Check sheet for the drawn part. Datum: minimum x, y, z corner. Units: mm. Round coordinates to 2 decimals unless told otherwise and drop trailing zeros. Order: outer loops, then holes, each group sorted by start corner. A loop starts at its lowest first (then second) coordinate and runs counter-clockwise, first axis right, second up. Notation, with made-up numbers: (-1, 7) -> (56, 7) arc R31 ccw to (56, 45) -> close; hole circle Ø4 at (30.5, -8.75). An arc over 180 degrees is marked (long way). Use CSV: the item, a comma, the result in double quotes.
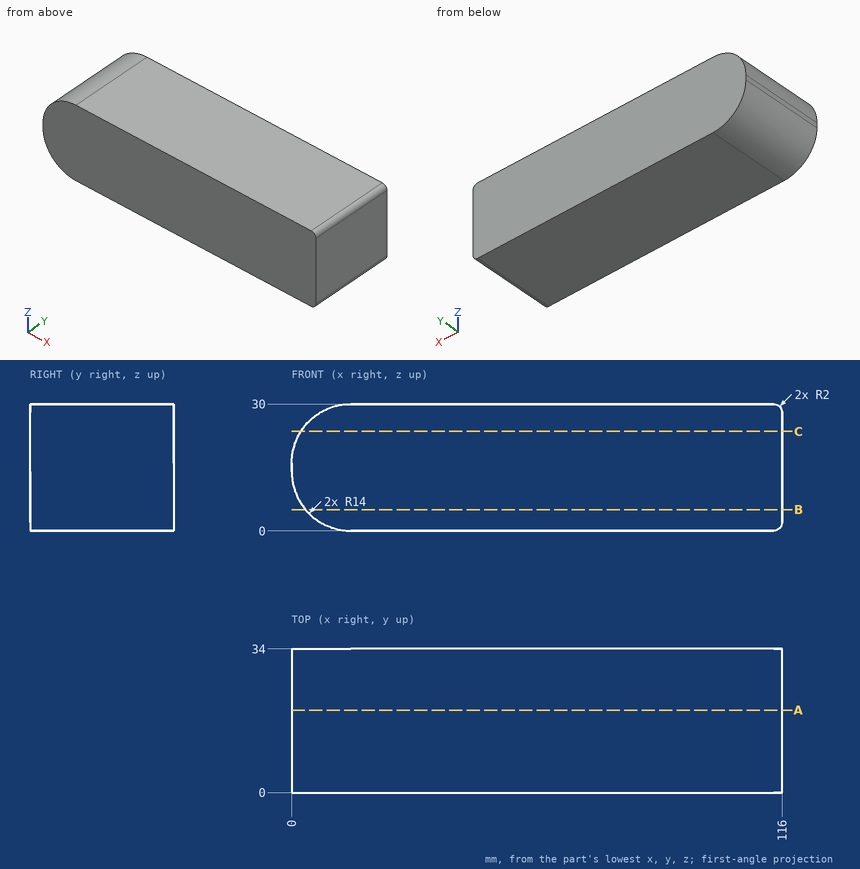
Q1. Scan lines: L1, parallel to X at y = 14.5, z = 17; L2, parallel to X at y = 12.5, z = 6; L3, parallel to Z at x = 10.5, y = 20.5. Record each from-to range of solid material in increasing order.
Result sheet:
L1,"x = 0.04 to 116"
L2,"x = 2.51 to 116"
L3,"z = 0.44 to 29.56"
Q2. Go/stop test with flat-tipped pins: pin 1 (4 mm diameter, centred on y = 12.5, z = 10.5, fed in from -X); pin 2 (4 mm diameter, centred on y = 25, z = 25, fed in from -X). Record where each tip stops, or that it passes through.
Result sheet:
pin 1,"stops at x = 0.08"
pin 2,"stops at x = 1.88"
Q3. Sectioned sample at A-A, the plane y = 19.5. Enter the section's corners in (x, z).
Result sheet:
outline,"(0, 14) arc R14 ccw to (14, 0) -> (114, 0) arc R2 ccw to (116, 2) -> (116, 28) arc R2 ccw to (114, 30) -> (14, 30) arc R14 ccw to (0, 16) -> close"
Q4. Sectioned sample at C-C, the plane z = 23.5. Enter the section's corners in (x, y).
Result sheet:
outline,"(2.18, 0) -> (116, 0) -> (116, 34) -> (2.18, 34) -> close"
Q5. Sectioned sample at B-B, the plane z = 5. Enter the section's corners in (x, y), then the cut area to 3 significant figures.
Result sheet:
outline,"(3.28, 0) -> (116, 0) -> (116, 34) -> (3.28, 34) -> close"
area,"3,830 mm^2"
